```python
from build123d import *

# Parameters (mm, degrees)
F0_R     = 2.5
F0_W     = 13.873467
F0_H     = 10.023556
F1_DEPTH = 2


with BuildPart() as f1:
    # F0 (on Front) → F1 (new body)
    with BuildSketch(Plane.XZ):
        with BuildLine():
            ThreePointArc((36.719143, 15.101325), (37.419231, 24.186519), (28.334037, 23.486431))
            ThreePointArc((28.334037, 23.486431), (13.17659, 27.943878), (-1.980857, 23.486431))
            ThreePointArc((-1.980857, 23.486431), (-7.144612, 25.935274), (-12.016955, 22.94839))
            Line((-12.016955, 22.94839), (-31.629865, 22.94839))
            ThreePointArc((-31.629865, 22.94839), (-36.502208, 25.935274), (-41.665963, 23.486431))
            ThreePointArc((-41.665963, 23.486431), (-56.82341, 27.943878), (-71.980857, 23.486431))
            ThreePointArc((-71.980857, 23.486431), (-81.066051, 24.186519), (-80.365963, 15.101325))
            ThreePointArc((-80.365963, 15.101325), (-84.82341, -0.056122), (-80.365963, -15.213569))
            ThreePointArc((-80.365963, -15.213569), (-81.066051, -24.298763), (-71.980857, -23.598675))
            ThreePointArc((-71.980857, -23.598675), (-56.82341, -28.056122), (-41.665963, -23.598675))
            ThreePointArc((-41.665963, -23.598675), (-36.502208, -26.047518), (-31.629865, -23.060634))
            Line((-31.629865, -23.060634), (-12.016955, -23.060634))
            ThreePointArc((-12.016955, -23.060634), (-7.144612, -26.047518), (-1.980857, -23.598675))
            ThreePointArc((-1.980857, -23.598675), (13.17659, -28.056122), (28.334037, -23.598675))
            ThreePointArc((28.334037, -23.598675), (37.419231, -24.298763), (36.719143, -15.213569))
            ThreePointArc((36.719143, -15.213569), (38.161421, -12.695672), (39.335368, -10.042029))
            ThreePointArc((39.335368, -10.042029), (41.668623, -2.730663), (41.24273, 4.932154))
            ThreePointArc((41.24273, 4.932154), (40.446435, 7.495779), (39.332206, 9.938063))
            ThreePointArc((39.332206, 9.938063), (38.159421, 12.587381), (36.719143, 15.101325))
        make_face()
        with Locations((-76.82341, -20.056122)):
            Circle(F0_R, mode=Mode.SUBTRACT)
        with Locations((-36.82341, -20.056122)):
            Circle(F0_R, mode=Mode.SUBTRACT)
        with BuildLine():
            ThreePointArc((-12.972297, -10.0679), (-11.801986, -12.708028), (-10.365963, -15.213569))
            ThreePointArc((-10.365963, -15.213569), (-11.639118, -16.477162), (-12.481857, -18.060634))
            Line((-12.481857, -18.060634), (-31.164963, -18.060634))
            ThreePointArc((-31.164963, -18.060634), (-32.007702, -16.477162), (-33.280857, -15.213569))
            ThreePointArc((-33.280857, -15.213569), (-31.844834, -12.708028), (-30.674523, -10.0679))
            Line((-30.674523, -10.0679), (-12.972297, -10.0679))
        make_face(mode=Mode.SUBTRACT)
        with BuildLine():
            ThreePointArc((-62.942122, 7.853453), (-65.800801, 4.349152), (-66.82341, -0.056122))
            ThreePointArc((-66.82341, -0.056122), (-66.823361, -0.080004), (-66.823296, -0.103885))
            ThreePointArc((-66.823296, -0.103885), (-64.289716, -12.78048), (-57.144925, -23.553922))
            ThreePointArc((-57.144925, -23.553922), (-72.940781, -17.158179), (-80.260911, -1.768888))
            ThreePointArc((-80.260911, -1.768888), (-72.36496, 4.416369), (-62.942122, 7.853453))
        make_face(mode=Mode.SUBTRACT)
        with BuildLine():
            ThreePointArc((-64.718322, -6.193741), (-61.217941, -9.038777), (-56.82341, -10.056122))
            ThreePointArc((-56.82341, -10.056122), (-44.12797, -7.557344), (-33.326445, -0.433782))
            ThreePointArc((-33.326445, -0.433782), (-39.721353, -16.173493), (-55.054649, -23.489463))
            ThreePointArc((-55.054649, -23.489463), (-61.25874, -15.608324), (-64.718322, -6.193741))
        make_face(mode=Mode.SUBTRACT)
        with Locations((-6.82341, -20.056122)):
            Circle(F0_R, mode=Mode.SUBTRACT)
        with Locations((33.17659, -20.056122)):
            Circle(F0_R, mode=Mode.SUBTRACT)
        with BuildLine():
            ThreePointArc((7.057878, 7.853453), (4.199459, 4.349684), (3.17659, -0.054937))
            ThreePointArc((3.17659, -0.054937), (3.176641, -0.080004), (3.17671, -0.10507))
            ThreePointArc((3.17671, -0.10507), (5.710512, -12.781028), (12.855078, -23.553922))
            ThreePointArc((12.855078, -23.553922), (-2.94078, -17.15818), (-10.260911, -1.768888))
            ThreePointArc((-10.260911, -1.768888), (-2.36496, 4.416369), (7.057878, 7.853453))
        make_face(mode=Mode.SUBTRACT)
        with BuildLine():
            ThreePointArc((5.281681, -6.193744), (8.782061, -9.038778), (13.17659, -10.056122))
            ThreePointArc((13.17659, -10.056122), (25.87203, -7.557344), (36.673555, -0.433782))
            ThreePointArc((36.673555, -0.433782), (30.278648, -16.173492), (14.945354, -23.489463))
            ThreePointArc((14.945354, -23.489463), (8.741263, -15.608326), (5.281681, -6.193744))
        make_face(mode=Mode.SUBTRACT)
        with BuildLine():
            ThreePointArc((-80.320375, 0.321538), (-73.9062, 16.081669), (-58.536176, 23.381379))
            ThreePointArc((-58.536176, 23.381379), (-52.350919, 15.485428), (-48.913835, 6.06259))
            ThreePointArc((-48.913835, 6.06259), (-52.418136, 8.92127), (-56.82341, 9.943878))
            ThreePointArc((-56.82341, 9.943878), (-69.51885, 7.445101), (-80.320375, 0.321538))
        make_face(mode=Mode.SUBTRACT)
        with Locations((-21.82341, -0.056122)):
            Rectangle(F0_W, F0_H, mode=Mode.SUBTRACT)
        with BuildLine():
            ThreePointArc((-50.704698, -7.965696), (-47.846018, -4.461396), (-46.82341, -0.056122))
            ThreePointArc((-46.82341, -0.056122), (-49.322187, 12.639318), (-56.44575, 23.440843))
            ThreePointArc((-56.44575, 23.440843), (-40.685619, 17.026668), (-33.385909, 1.656644))
            ThreePointArc((-33.385909, 1.656644), (-41.28186, -4.528612), (-50.704698, -7.965696))
        make_face(mode=Mode.SUBTRACT)
        with Locations((-76.82341, 19.943878)):
            Circle(F0_R, mode=Mode.SUBTRACT)
        with BuildLine():
            Line((-12.972297, 9.955656), (-30.674523, 9.955656))
            ThreePointArc((-30.674523, 9.955656), (-31.844834, 12.595784), (-33.280857, 15.101325))
            ThreePointArc((-33.280857, 15.101325), (-32.007702, 16.364918), (-31.164963, 17.94839))
            Line((-31.164963, 17.94839), (-12.481857, 17.94839))
            ThreePointArc((-12.481857, 17.94839), (-11.639118, 16.364918), (-10.365963, 15.101325))
            ThreePointArc((-10.365963, 15.101325), (-11.801986, 12.595784), (-12.972297, 9.955656))
        make_face(mode=Mode.SUBTRACT)
        with Locations((-36.82341, 19.943878)):
            Circle(F0_R, mode=Mode.SUBTRACT)
        with BuildLine():
            ThreePointArc((-10.320375, 0.321538), (-3.905793, 16.082099), (11.465005, 23.381465))
            ThreePointArc((11.465005, 23.381465), (17.649864, 15.485203), (21.086473, 6.062191))
            ThreePointArc((21.086473, 6.062191), (17.582091, 8.921159), (13.17659, 9.943878))
            ThreePointArc((13.17659, 9.943878), (0.48115, 7.445101), (-10.320375, 0.321538))
        make_face(mode=Mode.SUBTRACT)
        with BuildLine():
            ThreePointArc((19.295302, -7.965696), (22.154242, -4.460865), (23.17659, -0.054937))
            ThreePointArc((23.17659, -0.054937), (20.678132, 12.639721), (13.555434, 23.440824))
            ThreePointArc((13.555434, 23.440824), (29.314811, 17.026261), (36.614091, 1.656644))
            ThreePointArc((36.614091, 1.656644), (28.71814, -4.528612), (19.295302, -7.965696))
        make_face(mode=Mode.SUBTRACT)
        with Locations((-6.82341, 19.943878)):
            Circle(F0_R, mode=Mode.SUBTRACT)
        with Locations((33.17659, 19.943878)):
            Circle(F0_R, mode=Mode.SUBTRACT)
    extrude(amount=F1_DEPTH)


with BuildPart() as f1_1:
    # F2: moved
    add(f1.part.moved(Location((21.6, 0, 0))))


solid = f1_1.part
```
The model under review builds one solid part; all positions refer to its coordinate system, in mm. A direction names the side the tool comes from. Round coordinates to 2 decimals unless told otherwise and drop trailing zeros. Loops run counter-clockwise (first coordinate to the right, second up) from the corner with the lowest first, then second, coordinate; pieces in that order, holes last. Notation, with made-up numbers: M -33.5,14 L 6.5,14 A7 ccw 6.5,27 Z; hole C 29.25,38 d7. An arc over 180 degrees is marked long. Answer as a JSON object with one key per item and string values.
(1) Clearance check with flat-ended pins moving along their axes: P1, Ø1, axis at x = 1, y = -1, coming from the -Z side; P2, Ø1, axis at x = 0, y = -1, coming from the +Z side. State where each tip first meets the part, or that it passes through.
Resolved:
{"P1": "z = -23.06", "P2": "z = 22.95"}
(2) Take a section at A-A on x = -0.5. Give the boundary of the cut face in (y, z), and give its area (3 significant figures).
Resolved:
{"outline": "M -2,-23.06 L 0,-23.06 L 0,-18.06 L -2,-18.06 Z; M -2,-10.07 L 0,-10.07 L 0,-5.07 L -2,-5.07 Z; M -2,4.96 L 0,4.96 L 0,9.96 L -2,9.96 Z; M -2,17.95 L 0,17.95 L 0,22.95 L -2,22.95 Z", "area": "40.0 mm²"}
(3) Take a section at C-C on x = -47. Give the boundary of the cut face in (y, z).
Resolved:
{"outline": "M -2,-25.46 L 0,-25.46 L 0,-20.39 L -2,-20.39 Z; M -2,6.2 L 0,6.2 L 0,7.81 L -2,7.81 Z; M -2,20.28 L 0,20.28 L 0,25.35 L -2,25.35 Z"}
(4) Take a section at B-B on z = -3. Count the separate pieces of the cut face and the enclosed holes in it, and give its area (3 significant figures).
Resolved:
{"separate pieces": "8", "enclosed holes": "0", "area": "126 mm²"}
(5) To check wall thickness, follow line 1 along Z through (x, y) = (-7.5, -1.7); line 2 along X through (y, z) = (-1.05, 13.5); line 3 along X through (y, z) = (-1.65, 15). State the ranges of each line that lie inside material, in increasing order.
Resolved:
{"line 1": "-23.06 to -18.06, -10.07 to 9.96, 17.95 to 22.95", "line 2": "-59.72 to -54.42, -29.74 to -28.09, -16.03 to -10.72, 10.28 to 15.58, 40.26 to 41.91, 53.97 to 59.28", "line 3": "-58.83 to -53.27, -30.49 to -28.8, -17.18 to -11.62, 11.17 to 16.73, 39.51 to 41.2, 52.82 to 58.38"}
(6) Draft analysis for pull direction Z (two halves, no side actions). For faces 3 (the cylindrical face through (-39.59, -0.99, -15.73)), 4 (the flat face through (-1, -2, -6)), 5 (the cylindrical face through (-14.82, -0.99, 25.93)), 6 (the cylindrical face through (17.528, -0.986, 15.904)), state which applies: released by +Z, released by -Z, zero draft, split by the parting line, or undercut.
Resolved:
{"face 3": "undercut", "face 4": "zero draft", "face 5": "released by +Z", "face 6": "undercut"}
(7) Tool access review of faces 1 (the flat face through (-1, 0, -6)), 2 (the cylindrical face through (9.976, -0.986, -16.457)): name each direction out of +Z, -Z, +X, -X, +Y, -Y from which nothing blocks a thin tool from reaching the whole face with its end or side.
Resolved:
{"face 1": "+Z, -Z, +X, -X, +Y", "face 2": "+Y, -Y"}
